Build history of the part. All positions in model axes, mm. A direction names the side the tool comes from. Round coordinates to 2 decimals unless told otherwise and drop trailing zeros. Write each loop counter-clockwise with the first axis right and the second up, starting at its lowest first coordinate (ties: lowest second). Pieces come first, ordered by that corner, then holes. Notation, with made-up numbers: (73, 46.5) - (91, 46.5) arc R26 cw to (91, 85.5) - close; hole circle Ø8 at (50, -6). An arc over 180 degrees is marked (long way). Answer as a JSON object with one key per item and string values. Group by question number.
Item 1: Slice it at A-A, the plane y = 6. List the corners of the cut face in (x, z), then the cut area to 3 significant figures.
Item 2: Flat gauge pins, fed straight in: pin 1 (1.5 mm diameter, centred on x = 51.5, z = -22, fed in from +Y); pin 2 (12 mm diameter, centred on x = 55.5, z = -28, fed in from -Y); pin 3 (1 mm diameter, centred on x = 50.5, z = -72, fed in from +Y). Where does each tip first touch, or does it go through?
Item 3: Slice it at D-D, the plane z = -59.5. List the corners of the cut face in (x, y), then the cut area to 3 significant figures.
Item 4: Slice it at B-B, the plane x = 31.5. List the corners of the cut face in (y, z), then the cut area to 3 significant figures.
Item 5: Two-plate mould, pull along Z, no slides. Class faces 3 (the flat face through (62.354, 10.078, -79.514)), 4 (the flat face through (60, 18, -32)): +Z half, -Z half, draft (parallel to the pull), parting line (faces both ways), or undercut.
Item 6: Which spindle directions (+Z, -Z, +X, -X, +Y, -Y) get a long thin tool onto all of the face, cutting with end or side? Do faces 1 (the flat face through (13, 16, -25)), 2 (the flat face through (72, 9, -41)). Say none if no direction does.
Item 7: Probe line 1 (Z direction, x = 41, y = 17.25); line 2 (Z direction, x = 27, y = 6.5); line 3 (X direction, y = 2.75, z = -53.5). List the from-to ranges inside material, lowest first. Write a range as from..to.
Item 8: Slice it at C-C, the plane z = -41.5. List the corners of the cut face in (x, y).
from build123d import *

# Parameters (mm, degrees)
SKETCH1_W           = 72
SKETCH1_H           = 83
BOSS_EXTRUDE1_DEPTH = 18
CAVITY2_START       = -80.5
CAVITY2_DEPTH       = 34
CAVITY2_START_2     = -48.5
CAVITY2_2_DEPTH     = 46
CAVITY2_3_DEPTH     = 5
CAVITY2_START_3     = -51.5
CAVITY2_4_DEPTH     = 5
CAVITY2_START_4     = -4.5
CAVITY2_5_OUTLINE_W = 37
CAVITY2_5_OUTLINE_H = 5
CAVITY2_5_DEPTH     = 2
CAVITY2_6_DEPTH     = 2
CAVITY2_7_DEPTH     = 2


# Read off the part's stored shape, not the designer's step: Cavity2
with BuildPart() as part:
    # Sketch1 → Boss-Extrude1 (new body)
    with BuildSketch(Plane(origin=(0, 0, 0), x_dir=(1, 0, 0), z_dir=(0, 1, 0))):
        with Locations((36, 41.5)):
            Rectangle(SKETCH1_W, SKETCH1_H)
    extrude(amount=BOSS_EXTRUDE1_DEPTH)

    # Cavity2 outline → Cavity2 (cut)
    with BuildSketch(Plane.XY.offset(CAVITY2_START)):
        Polygon((55.404610688, 2), (55.404610688, 12.86969785), (69.5, 18), (46.804610688, 18), (46.804610688, 2), align=None)
        Polygon((25.804610688, 18), (3.109221376, 18), (17.204610688, 12.86969785), (17.204610688, 2), (25.804610688, 2), align=None)
    extrude(amount=CAVITY2_DEPTH, mode=Mode.SUBTRACT)

    # Cavity2 2 outline → Cavity2 2 (cut)
    with BuildSketch(Plane.XY.offset(CAVITY2_START_2)):
        Polygon((55.404610688, 11), (57.404610688, 11), (57.404610688, 18), (8.404610688, 18), (8.404610688, 11), (10.404610688, 11), (10.404610688, 16), (16.404610688, 16), (16.404610688, 11), (18.404610688, 11), (18.404610688, 16), (55.404610688, 16), align=None)
    extrude(amount=CAVITY2_2_DEPTH, mode=Mode.SUBTRACT)

    # Cavity2 3 outline → Cavity2 3 (cut)
    with BuildSketch(Plane.XY.offset(CAVITY2_START)):
        Polygon((46.804610688, 2), (46.804610688, 18), (25.804610688, 18), (25.804610688, 2), (28.554610688, 2), (28.554610688, 16), (32.554610688, 16), (32.554610688, 2), align=None)
    extrude(amount=CAVITY2_3_DEPTH, mode=Mode.SUBTRACT)

    # Cavity2 4 outline → Cavity2 4 (cut)
    with BuildSketch(Plane.XY.offset(CAVITY2_START_3)):
        Polygon((46.804610688, 2), (46.804610688, 18), (25.804610688, 18), (25.804610688, 2), (40.054610688, 2), (40.054610688, 16), (44.054610688, 16), (44.054610688, 2), align=None)
    extrude(amount=CAVITY2_4_DEPTH, mode=Mode.SUBTRACT)

    # Cavity2 5 outline → Cavity2 5 (cut)
    with BuildSketch(Plane.XY.offset(CAVITY2_START_4)):
        with Locations((36.904610688, 13.5)):
            Rectangle(CAVITY2_5_OUTLINE_W, CAVITY2_5_OUTLINE_H)
    extrude(amount=CAVITY2_5_DEPTH, mode=Mode.SUBTRACT)

    # Cavity2 6 outline → Cavity2 6 (cut)
    with BuildSketch(Plane.XY.offset(CAVITY2_START)):
        Polygon((55.404610688, 7.548808988), (69.5, 12.679111138), (69.5, 18), (55.404610688, 12.86969785), align=None)
        Polygon((3.109221376, 18), (3.109221376, 12.679111138), (17.204610688, 7.548808988), (17.204610688, 12.86969785), align=None)
    extrude(amount=CAVITY2_6_DEPTH, mode=Mode.SUBTRACT)

    # Cavity2 7 outline → Cavity2 7 (cut)
    with BuildSketch(Plane.XY.offset(CAVITY2_START_2)):
        Polygon((55.404610688, 7.548808988), (69.5, 12.679111138), (69.5, 18), (57.404610688, 13.597638319), (57.404610688, 11), (55.404610688, 11), align=None)
        Polygon((8.404610688, 11), (8.404610688, 16.072635912), (3.109221376, 18), (3.109221376, 12.679111138), (17.204610688, 7.548808988), (17.204610688, 11), (16.404610688, 11), (16.404610688, 13.160874037), (10.404610688, 15.344695443), (10.404610688, 11), align=None)
    extrude(amount=CAVITY2_7_DEPTH, mode=Mode.SUBTRACT)


solid = part.part
Geometry says:
{
 "1": {"outline": "(0, -83) - (72, -83) - (72, 0) - (0, 0) - close; hole (17.2, -80.5) - (28.55, -80.5) - (28.55, -75.5) - (25.8, -75.5) - (25.8, -51.5) - (40.05, -51.5) - (40.05, -46.5) - (17.2, -46.5) - close; hole (32.55, -80.5) - (55.4, -80.5) - (55.4, -46.5) - (44.05, -46.5) - (44.05, -51.5) - (46.8, -51.5) - (46.8, -75.5) - (32.55, -75.5) - close", "area": "5,220 mm^2"},
 "2": {"pin 1": "stops at y = 16", "pin 2": "stops at y = 0", "pin 3": "stops at y = 2"},
 "3": {"outline": "(0, 0) - (72, 0) - (72, 18) - (69.5, 18) - (55.4, 12.87) - (55.4, 2) - (46.8, 2) - (46.8, 18) - (25.8, 18) - (25.8, 2) - (17.2, 2) - (17.2, 12.87) - (3.11, 18) - (0, 18) - close", "area": "948 mm^2"},
 "4": {"outline": "(0, -83) - (18, -83) - (18, -80.5) - (16, -80.5) - (16, -75.5) - (18, -75.5) - (18, -51.5) - (2, -51.5) - (2, -46.5) - (16, -46.5) - (16, -4.5) - (11, -4.5) - (11, -2.5) - (18, -2.5) - (18, 0) - (0, 0) - close", "area": "1,310 mm^2"},
 "5": {"face 3": "undercut", "face 4": "draft"},
 "6": {"face 1": "+Y", "face 2": "+Z, -Z, +X, +Y, -Y"},
 "7": {"line 1": "z = -83..-80.5, -75.5..-51.5, -2.5..0", "line 2": "z = -83..-80.5, -75.5..-51.5, -46.5..0", "line 3": "x = 0..17.2, 25.8..46.8, 55.4..72"},
 "8": {"outline": "(0, 0) - (72, 0) - (72, 18) - (57.4, 18) - (57.4, 11) - (55.4, 11) - (55.4, 16) - (18.4, 16) - (18.4, 11) - (16.4, 11) - (16.4, 16) - (10.4, 16) - (10.4, 11) - (8.4, 11) - (8.4, 18) - (0, 18) - close"}
}
